The model under review builds one solid part; all positions refer to its coordinate system, in mm. A direction names the side the tool comes from. Coordinates: 2 decimals unless noted, no trailing zeros. Order: outer loops, then holes, each group sorted by start corner. A loop starts at its lowest first (then second) coordinate and runs counter-clockwise, first axis right, second up. Notation, with made-up numbers: (-33.5, -22) -> (9.5, -22) arc R16 ccw to (9.5, -7) -> close; hole circle Ø11 at (45, 58). An arc over 180 degrees is marked (long way). Put each result on its own line as item: value.
from build123d import *

# Parameters (mm, degrees)
F1_DEPTH = 25.4
F3_DEPTH = 12.7
F5_DEPTH = 12.7
F7_DEPTH = 12.7


with BuildPart() as f1:
    # F0 (on Top) → F1 (new body)
    with BuildSketch(Plane.XY):
        Polygon((0, 38.1), (0, 0), (12.7, 0), (12.7, 38.1), (25.4, 38.1), (25.4, 69.85), (-12.7, 69.85), (-12.7, 38.1), align=None)
    extrude(amount=F1_DEPTH)

    # F2 (on face) → F3 (cut)
    with BuildSketch(Plane(origin=(-12.7, 0, 0), x_dir=(0, -1, 0), z_dir=(-1, 0, 0))):
        Polygon((-50.8, 25.4), (-38.1, 0), (-38.1, 25.4), align=None)
    extrude(amount=-F3_DEPTH, mode=Mode.SUBTRACT)

    # F4 (on face) → F5 (cut)
    with BuildSketch(Plane.YZ.offset(25.4)):
        Polygon((50.8, 25.4), (38.1, 25.4), (38.1, 0), align=None)
    extrude(amount=-F5_DEPTH, mode=Mode.SUBTRACT)

    # F6 (on face) → F7 (cut)
    with BuildSketch(Plane.YZ.offset(12.7)):
        Polygon((12.7, 25.4), (0, 25.4), (0, 0), align=None)
    extrude(amount=-F7_DEPTH, mode=Mode.SUBTRACT)


solid = f1.part
Item 1: Consider section C-C on x = -1.5. Write out the cut boundary in (y, z).
Answers below:
outline: (38.1, 0) -> (69.85, 0) -> (69.85, 25.4) -> (50.8, 25.4) -> close
Item 2: For faces 1 (the flat face through (12.7, 25, 13)), 2 (the flat face through (0, 26, 13)), 3 (the flat face through (6.44, 6.26, 12.52)), list the 3-axis set-ups (+Z, -Z, +X, -X, +Y, -Y) from which the entire face can be reached by the end or side of a thin tool; tool diameter is ignored.
Answers below:
face 1: +Z, +X, -Y
face 2: +Z, -X, -Y
face 3: +Z, +X, -X, -Y
Item 3: Consider section A-A on y = 50. Write out the cut boundary in (x, z), and give its area (3 significant figures).
Answers below:
outline: (-12.7, 0) -> (25.4, 0) -> (25.4, 23.8) -> (12.7, 23.8) -> (12.7, 25.4) -> (0, 25.4) -> (0, 23.8) -> (-12.7, 23.8) -> close
area: 927 mm^2
Item 4: For line 1 (X direction, y = 14, z = 4.5); line 2 (Z direction, x = -5, y = 43); line 3 (Y direction, x = 21, z = 21), list the stretches that pass through material, from the lowest coordinate up. Write a range as from..to.
Answers below:
line 1: 0..12.7
line 2: 0..9.8
line 3: 48.6..69.85
Item 5: For pin 1 Ø7.5 at (y, z) = (31, 16.5) entering from -X; pin 2 Ø2 at (x, z) = (21, 7.5) entering from -Y, all flat-tipped, find the tip position at first contact; note any pin that passes through.
Answers below:
pin 1: x = 0
pin 2: y = 41.35
Item 6: Consider section B-B on z = 3. Write out the cut boundary in (x, y).
Answers below:
outline: (-12.7, 39.6) -> (0, 39.6) -> (0, 1.5) -> (12.7, 1.5) -> (12.7, 39.6) -> (25.4, 39.6) -> (25.4, 69.85) -> (-12.7, 69.85) -> close
Item 7: Consider section D-D on y = 26.5. Write out the cut boundary in (x, z).
Answers below:
outline: (0, 0) -> (12.7, 0) -> (12.7, 25.4) -> (0, 25.4) -> close
